For this review, take the finished solid that the model builds, in its own axes (mm). A direction names the side the tool comes from. Give positions to 0.01 mm unless a question says otherwise; leave off trailing zeros. Write each loop counter-clockwise with the first axis right and the second up, starting at its lowest first coordinate (ties: lowest second). Pieces come first, ordered by that corner, then holes. Notation, with made-up numbers: M -29,57 L -8,57 A28 cw -8,75 Z; hole C -26,65 d1. An arc over 180 degrees is marked long. One line per item, written item: value. Start each with the question number.
Item 1: Consider section D-D, the plane x = 30. Write out the cut boundary in (y, z), and give its area (3 significant figures).
Item 2: Consider section A-A, the plane x = 108.5. Write out the cut boundary in (y, z).
Item 3: Clearance check with flat-ended pins moving along their axes: pin 1 Ø6 at (x, y) = (38, 56) entering from -Z; pin 2 Ø6 at (x, z) = (229, 222) entering from -Y; pin 3 Ø8 at (x, z) = (56.5, 208.5) entering from -Y; pin 4 Ø1.3 at (y, z) = (-223, -31.5) entering from -X. State where each tip first meets the part, or that it passes through.
Item 4: Mouldability with a two-part tool opening along Z and no side actions: class faces 4 (the face through (140.65, -300.128, 294.959)), 5 (the face through (1.288, -130.355, 79.057)), 6 (the face through (60.53, 220.33, 316.37)) as released by +Z, released by -Z, zero draft, split by the parting line, or undercut.
Item 5: Consider section C-C, the plane y = 39.5. Write out the cut boundary in (x, z), and give its area (3 significant figures).
Item 6: Tool access review of faces 1 (the face through (182, -224.409, -119)), 2 (the face through (141.25, -297.405, 293.917)), 3 (the face through (1.288, 104.21, 77.705)): name each direction out of +Z, -Z, +X, -X, +Y, -Y from which nothing blocks a thin tool from reaching the whole face with its end or side.
Item 7: Consider section B-B, the plane z = 63. Write out the cut boundary in (x, y).
Item 8: To check wall thickness, follow probe 1 along X at (y, z) = (-104, 159); probe 2 along X at (y, z) = (111, 19); probe 3 along Y at (x, z) = (151, -175). State the ranges of each line that lie inside material, in increasing order.
```python
from build123d import *

# Parameters (mm, degrees)
F1_DEPTH  = 368.3
F2_T      = -2.54
F3_W      = 241.3
F3_H      = 444.5
F4_DEPTH  = 25.4
F5_W      = 241.3
F5_H      = 266.7
F6_DEPTH  = 25.4
F7_W      = 241.3
F7_H      = 114.3
F8_DEPTH  = 25.4
F10_DEPTH = 25.4


with BuildPart() as f1:
    # F0 (on Right) → F1 (new body)
    with BuildSketch(Plane.YZ):
        Polygon((-224.4092495818, -219.5814980744), (169.2907504182, -219.5814980744), (413.1046041976, 226.0851988026), (-90.0800447439, 469.1132816853), (-344.2729837605, 258.357523154), (-224.4092495818, 34.4185019256), align=None)
    extrude(amount=F1_DEPTH)

    # F2
    f2_openings = [f1.faces().sort_by_distance(p)[0] for p in [
        (184.15, 291.197677, 3.25185),
        (184.15, -27.55925, -219.581498),
    ]]
    offset(amount=F2_T, openings=f2_openings, kind=Kind.INTERSECTION)

    # F3 (on face) → F4 (cut)
    with BuildSketch(Plane(origin=(0, 166.6783638091, 345.1041253529), x_dir=(1, 0, 0), z_dir=(0, 0.4349106709, 0.9004736023))):
        with Locations((184.15, -62.8870744342)):
            Rectangle(F3_W, F3_H)
    extrude(amount=-F4_DEPTH, mode=Mode.SUBTRACT)

    # F5 (on face) → F6 (cut)
    with BuildSketch(Plane(origin=(0, -267.194897424, 322.2642965476), x_dir=(1, 0, 0), z_dir=(0, -0.6382669853, 0.7698150788))):
        with Locations((184.15, 96.7245433025)):
            Rectangle(F5_W, F5_H)
    extrude(amount=-F6_DEPTH, mode=Mode.SUBTRACT)

    # F7 (on face) → F8 (cut)
    with BuildSketch(Plane.XZ.offset(224.4092495818)):
        with Locations((184.15, -35.4314980744)):
            Rectangle(F7_W, F7_H)
    extrude(amount=-F8_DEPTH, mode=Mode.SUBTRACT)

    # F9 (on face) → F10 (cut)
    with BuildSketch(Plane.YZ.offset(2.54)):
        with BuildLine():
            ThreePointArc((-98.6126363277, 46.6085672379), (85.2821775, 15.4665672824), (248.5302528965, -74.7398215894))
            Line((248.5302528965, -74.7398215894), (279.006984619, -19.0314844798))
            ThreePointArc((279.006984619, -19.0314844798), (101.5154343461, 78.6343708282), (-98.6126363277, 110.1085672379))
            ThreePointArc((-98.6126363277, 110.1085672379), (-130.3626363277, 78.3585672379), (-98.6126363277, 46.6085672379))
        make_face()
    extrude(amount=-F10_DEPTH, mode=Mode.SUBTRACT)


solid = f1.part
```
Model answer:
1. outline: M -344.27,258.36 L -224.41,34.42 L -224.41,-219.58 L -221.87,-219.58 L -221.87,35.06 L -341.05,257.73 L -89.72,466.12 L 411.88,223.85 L 413.1,226.09 L -90.08,469.11 Z
1. area: 3,540 mm2
2. outline: M -344.27,258.36 L -224.41,34.42 L -224.41,21.72 L -221.87,21.72 L -221.87,35.06 L -341.05,257.73 L -293.77,296.93 L -295.39,298.89 Z; M -224.41,-219.58 L -221.87,-219.58 L -221.87,-92.58 L -224.41,-92.58 Z; M 309.08,273.51 L 411.88,223.85 L 413.1,226.09 L 310.18,275.8 Z
3. pin 1: stops at z = 394.29
3. pin 2: stops at y = -326.42
3. pin 3: stops at y = -319.73
3. pin 4: stops at x = 0
4. face 4: released by +Z
4. face 5: undercut
4. face 6: released by -Z
5. outline: M 0,-219.58 L 2.54,-219.58 L 2.54,29.29 L 0,29.29 Z; M 0,96.1 L 2.54,96.1 L 2.54,403.71 L 63.5,403.71 L 63.5,406.53 L 0,406.53 Z; M 304.8,403.71 L 365.76,403.71 L 365.76,-219.58 L 368.3,-219.58 L 368.3,406.53 L 304.8,406.53 Z
5. area: 3,350 mm2
6. face 1: -Z, +X, -X, -Y
6. face 2: none
6. face 3: -X
7. outline: M 0,-239.71 L 368.3,-239.71 L 368.3,323.88 L 365.76,323.88 L 365.76,-236.83 L 2.54,-236.83 L 2.54,-126.4 L 0,-126.4 Z; M 0,142.22 L 2.54,142.22 L 2.54,323.88 L 0,323.88 Z
8. probe 1: x = 0 to 2.54, 365.76 to 368.3
8. probe 2: x = 365.76 to 368.3
8. probe 3: y = -224.41 to -221.87
